Can you work these out from the model? Positions are in its coordinate system, mm. A direction names the side the tool comes from. Give positions to 0.01 mm unless a question says otherwise; leave off trailing zeros. Write each loop counter-clockwise with the first axis right and the second up, starting at its lowest first coordinate (ties: lowest second). Pieces come first, ordered by that corner, then holes.
Autodesk Inventor part; units mm, degrees
ref_plane "YZ Plane" through (0, 0, 0) normal (1, 0, 0) x (0, 1, 0)
ref_plane "XZ Plane" through (0, 0, 0) normal (0, 1, 0) x (-1, 0, 0)
ref_plane "XY Plane" through (0, 0, 0) normal (0, 0, 1) x (1, 0, 0)
sketch "Sketch1" plane through (0, 0, 0) normal (0, 0, 1) x (1, 0, 0)
  line L0 (-50, 50) -> (50, 50)
  line L1 (50, 50) -> (50, -50)
  line L2 (50, -50) -> (-50, -50)
  line L3 (-50, -50) -> (-50, 50)
  line L4 (-50, 50) -> (50, -50) construction
  line L5 (50, 50) -> (-50, -50) construction
  point P0 (0, 0)
  dimension "d0" = 100
  dimension "d1" = 100
extrude "Extrusion1" add sketch "Sketch1" along normal blind 1500
sketch "Sketch2" plane through (0, 0, 1500) normal (0, 0, 1) x (1, 0, 0)
  line L0 (-40, 40) -> (40, 40)
  line L1 (40, 40) -> (40, -40)
  line L2 (40, -40) -> (-40, -40)
  line L3 (-40, -40) -> (-40, 40)
  line L4 (-40, 40) -> (40, -40) construction
  line L5 (40, 40) -> (-40, -40) construction
  point P0 (0, 0)
  dimension "d4" = 80
  dimension "d5" = 80
extrude "Extrusion2" cut sketch "Sketch2" against normal blind 1500
sketch "Sketch3" plane through (50, -50, 0) normal (1, 0, 0) x (0, 0, -1)
  line L0 (0, 100) -> (0, 0)
  circle A0 centre (-350, 50) radius 25
  circle A1 centre (-500, 50) radius 25
  circle A2 centre (-650, 50) radius 25
  circle A3 centre (-800, 50) radius 25
  point P0 (0, 50)
  dimension "d8" = 50
  dimension "d9" = 50
  dimension "d10" = 50
  dimension "d11" = 50
  dimension "d12" = 350
  dimension "d13" = 150
  dimension "d14" = 150
  dimension "d15" = 150
extrude "Extrusion3" cut sketch "Sketch3" against normal blind 1000
properties part number "atas 2"
(1) If I drill on L1, parallel to X at y = -15, z = 1075.5; L2, parallel to Y at x = -47.75, z = 500, over which ranges is the centre line in solid material (lowest first)?
Returned:
L1: x = -50 to -40, 40 to 50
L2: y = -50 to -25, 25 to 50
(2) Imagine slicing it at B-B, the plane x = 2. Write out the boundary of the cut face in (y, z).
Returned:
outline: (-50, 0) - (-40, 0) - (-40, 1500) - (-50, 1500) - close; (40, 0) - (50, 0) - (50, 1500) - (40, 1500) - close
(3) Imagine slicing it at A-A, the plane z = 105. Write out the boundary of the cut face in (x, y).
Returned:
outline: (-50, -50) - (50, -50) - (50, 50) - (-50, 50) - close; hole (-40, -40) - (40, -40) - (40, 40) - (-40, 40) - close
(4) If we mould it in two halves opening along Z, with no side actions, what happens to faces 1 (the face through (-44.93, 7.509, 626.154)), 2 (the face through (-45, 1, 0)), 3 (the face through (-1, 50, 740))? For each: +Z half, -Z half, draft (parallel to the pull), parting line (faces both ways), or undercut.
Returned:
face 1: undercut
face 2: -Z half
face 3: draft
(5) Imagine slicing it at D-D, the plane y = 0. Give the number of separate pieces and of enclosed holes in the cut face, plus the area to 3 significant figures.
Returned:
separate pieces: 10
enclosed holes: 0
area: 26,000 mm2
(6) Imagine slicing it at C-C, the plane z = 500. Write out the boundary of the cut face in (x, y), plus the area to 3 significant figures.
Returned:
outline: (-50, -50) - (50, -50) - (50, -25) - (40, -25) - (40, -40) - (-40, -40) - (-40, -25) - (-50, -25) - close; (-50, 25) - (-40, 25) - (-40, 40) - (40, 40) - (40, 25) - (50, 25) - (50, 50) - (-50, 50) - close
area: 2,600 mm2
(7) For faces 4 (the face through (50, 1, 740)), 5 (the face through (-1, 40, 760)), which set-ups out of +Z, -Z, +X, -X, +Y, -Y let a thin tool reach every point of the face, with its end or its side?
Returned:
face 4: +Z, -Z, +X, +Y, -Y
face 5: +Z, -Z
